Here's how the part is built. I have some questions about the finished solid (model axes, mm). A direction names the side the tool comes from. Round coordinates to 2 decimals unless told otherwise and drop trailing zeros. Order: outer loops, then holes, each group sorted by start corner. A loop starts at its lowest first (then second) coordinate and runs counter-clockwise, first axis right, second up. Notation, with made-up numbers: (1.25, 11.25) -> (7.25, 11.25) arc R11 ccw to (7.25, 31.25) -> close; hole circle Ø6 at (-27, 30). An arc over 180 degrees is marked (long way). Use a Markdown table: item, result. Add a question column.
(1) Thinking about a two-plate mould opening in Z: for faces 1 (the face through (-0.867, -3.905, 24.294)), 2 (the face through (-1.73, -7.81, 31.66)), which applies, pulls with the +Z half, pulls with the -Z half, needs draft (parallel to the pull), parting line crosses it, or undercut?
(2) I want a section at A-A, the plane z = 7. Please give me the cut outline in (x, y).
(3) I'm going to push flat-ended pins straight in: P1, Ø5, axis at y = 3, z = 17, coming from the -X side; P2, Ø12, axis at x = 9, z = 13, coming from the -Y side; P3, Ø2, axis at x = -2, z = 11.5, coming from the +Y side. Where does each tip first touch, or does it pass through?
(4) On a 3-axis mill with a long thin cutter (end or side, diameter ignored), from which of +Z, -Z, +X, -X, +Y, -Y can I reach the whole of each face in a straight line? I mean faces 3 (the face through (0, -5, 19.78)), 4 (the face through (5.19, -9.98, 15.54)). Say none if no direction works.
(5) I want a section at B-B, the plane y = -5.25. Give the number of separate pieces and of enclosed holes in the cut face, then the cut area to 3 significant figures.
(6) If I drill on probe 1 along Y at (x, z) = (0, 31.5); probe 2 along Y at (x, z) = (0, 22.5); probe 3 along X at (y, z) = (-5.75, 26), over which ranges is the centre line in solid material (lowest first)?
from build123d import *

# Parameters (mm, degrees)
F2_W = 11.213089
F2_H = 2


with BuildPart() as f1:
    # F0 (on Front) → F1 (revolve)
    with BuildSketch(Plane.XZ):
        Polygon((2.6, 42.62), (2.6, 0), (11.25, 0), (11.25, 26.28), (4.48, 26.28), (4.48, 27.77), (8, 27.77), (8, 28.77), (4.8, 28.77), (4.8, 30.21), (8, 30.21), (8, 33.07), (6, 33.07), (6, 38.97), (8, 38.97), (8, 42.62), align=None)
    revolve(axis=Axis((0, 0, 5.449006), (0, 0, 1)))

    # F2 (on Front) → F3 (revolve, cut)
    with BuildSketch(Plane.XZ):
        with Locations((9.606545, -3.72)):
            Rectangle(F2_W, F2_H)
        with Locations((9.606545, -0.22)):
            Rectangle(F2_W, F2_H)
        with Locations((9.606545, 3.28)):
            Rectangle(F2_W, F2_H)
        with Locations((9.606545, 6.78)):
            Rectangle(F2_W, F2_H)
        with Locations((9.606545, 10.28)):
            Rectangle(F2_W, F2_H)
        with Locations((9.606545, 13.78)):
            Rectangle(F2_W, F2_H)
        with Locations((9.606545, 17.28)):
            Rectangle(F2_W, F2_H)
        with Locations((9.606545, 20.78)):
            Rectangle(F2_W, F2_H)
        with Locations((9.606545, 24.28)):
            Rectangle(F2_W, F2_H)
    revolve(axis=Axis((0, 0, 3.329653), (0, 0, 1)), mode=Mode.SUBTRACT)


solid = f1.part
Taken from the geometry:
| question | item | result |
|---|---|---|
| 1 | face 1 | undercut |
| 1 | face 2 | needs draft |
| 2 | outline | circle Ø8 at (0, 0); hole circle Ø5.2 at (0, 0) |
| 3 | P1 | stops at x = -11.23 |
| 3 | P2 | stops at y = -10.84 |
| 3 | P3 | stops at y = 11.21 |
| 4 | face 3 | none |
| 4 | face 4 | +Z, -Z |
| 5 | separate pieces | 10 |
| 5 | enclosed holes | 0 |
| 5 | area | 354 mm2 |
| 6 | probe 1 | y = -8 to -2.6, 2.6 to 8 |
| 6 | probe 2 | y = -11.25 to -2.6, 2.6 to 11.25 |
| 6 | probe 3 | x = -9.67 to 9.67 |
